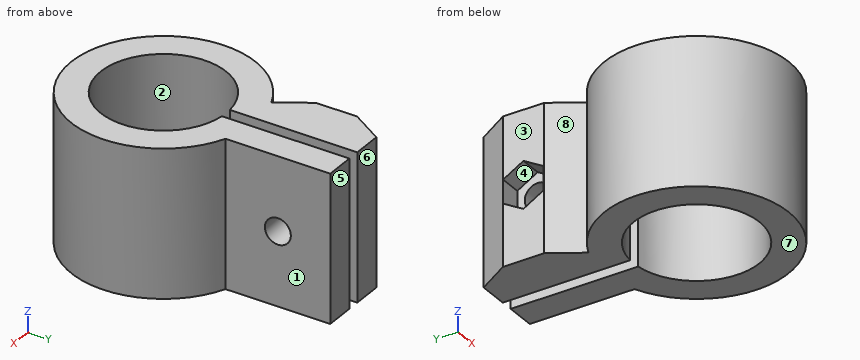
```python
from build123d import *

# Parameters (mm, degrees)
F1_DEPTH = 30
F3_DEPTH = 4.5
F4_R     = 2.646799
F5_DEPTH = 25.551


with BuildPart() as f1:
    # F0 (on Top) → F1 (new body)
    with BuildSketch(Plane.XY):
        with BuildLine():
            ThreePointArc((1.25, 12.738819), (0, -12.8), (-1.25, 12.738819))
            Line((-1.25, 12.738819), (-1.25, 38.745821))
            Line((-1.25, 38.745821), (-7.25, 38.745821))
            Line((-7.25, 38.745821), (-7.25, 17.345821))
            ThreePointArc((-7.25, 17.345821), (0, -18.8), (7.25, 17.345821))
            Line((7.25, 17.345821), (7.25, 38.738819))
            Line((7.25, 38.738819), (1.25, 38.738819))
            Line((1.25, 38.738819), (1.25, 12.738819))
        make_face()
        Polygon((-7.25, 17.345821), (-7.25, 38.745821), (-11.25, 32.245821), (-11.25, 23.845821), align=None)
    extrude(amount=F1_DEPTH)

    # F2 (on face) → F3 (cut)
    with BuildSketch(Plane(origin=(-11.25, 0, 0), x_dir=(0, -1, 0), z_dir=(-1, 0, 0))):
        Polygon((-32.195821, 17.396004), (-32.195821, 12.603996), (-28.045821, 10.207993), (-23.895821, 12.603996), (-23.895821, 17.396004), (-28.045821, 19.792007), align=None)
    extrude(amount=-F3_DEPTH, mode=Mode.SUBTRACT)

    # F4 (on face) → F5 (cut, through all)
    with BuildSketch(Plane(origin=(-6.75, 0, 0), x_dir=(0, -1, 0), z_dir=(-1, 0, 0))):
        with Locations((-28.045821, 15)):
            Circle(F4_R)
    extrude(amount=-F5_DEPTH, mode=Mode.SUBTRACT)


solid = f1.part
```
Geometry: final body of the model. Coordinates: model frame, mm. Face numbers are marked on the shaded views. A direction names the side the tool comes from. Round coordinates to 2 decimals unless told otherwise and drop trailing zeros. Loops run counter-clockwise (first coordinate to the right, second up) from the corner with the lowest first, then second, coordinate; pieces in that order, holes last. Notation, with made-up numbers: (-18.5, -22.5) -> (28.5, -22.5) arc R20 ccw to (28.5, -10.5) -> close; hole circle Ø7 at (-31, 67). An arc over 180 degrees is marked (long way). Use one line per item in the form item = value. Start each with the question number.
1) First-contact query: P1, Ø12, axis at x = 5.5, y = 24, coming from the -Z side; P2, Ø3, axis at x = -15, z = 19.5, coming from the -Y side; P3, Ø6.5, axis at y = 23.5, z = 13, coming from the +X side; P4, Ø1.5, axis at y = -7, z = 25.5, coming from the -X side. Flat tips, straight axial feed; report the tip coordinate or a pass-through.
2) Draft query along Y for the marked faces 6, 7 and 8. Return one class per face: released by +Y, released by -Y, zero draft, split by the parting line, or undercut.
3) Access query for the marked faces 1, 2, 3, 4 and 5. Directions: +Z, -Z, +X, -X, +Y, -Y. A direction counts if a zero-diameter tool reaches every point of the face in a straight line with its end or side. Return the directions, or none.
4) Section A-A on y = 0. Output: boundary loops of the cut face in (x, z).
5) Line query: L1, parallel to X at y = 27, z = 10; L2, parallel to X at y = 0, z = 13; L3, parallel to Y at x = -9, z = 25.25. Output: solid intervals per line, ascending.
6) Section D-D on x = 11.5. Output: boundary loops of the cut face in (y, z), then the cut area to 3 significant figures.
7) Section C-C on z = 15. Output: boundary loops of the cut face in (x, y), then the cut area to 3 significant figures.
8) Section B-B on x = -6. Output: boundary loops of the cut face in (y, z), then the cut area to 3 significant figures.
Response:
q1.P1 = 0
q1.P2 = -13.08
q1.P3 = 7.25
q1.P4 = -17.73
q2.face_6 = released by +Y
q2.face_7 = zero draft
q2.face_8 = undercut
q3.face_1 = +Z, -Z, +X, +Y
q3.face_2 = +Z, -Z
q3.face_3 = +Z, -Z, -X, +Y
q3.face_4 = -X
q3.face_5 = +Z, -Z, +X, -X, +Y
q4.outline = (-18.8, 0) -> (-12.8, 0) -> (-12.8, 30) -> (-18.8, 30) -> close; (12.8, 0) -> (18.8, 0) -> (18.8, 30) -> (12.8, 30) -> close
q5.L1 = -11.25 to -1.25, 1.25 to 7.25
q5.L2 = -18.8 to -12.8, 12.8 to 18.8
q5.L3 = -16.51 to -9.1, 9.1 to 16.51, 20.19 to 35.9
q6.outline = (-14.87, 0) -> (-5.62, 0) -> (-5.62, 30) -> (-14.87, 30) -> close; (5.62, 0) -> (14.87, 0) -> (14.87, 30) -> (5.62, 30) -> close
q6.area = 555 mm^2
q7.outline = (-11.25, 23.85) -> (-7.25, 17.35) arc R18.8 ccw (long way) to (7.25, 17.35) -> (7.25, 25.4) -> (1.25, 25.4) -> (1.25, 12.74) arc R12.8 cw (long way) to (-1.25, 12.74) -> (-1.25, 25.4) -> (-6.75, 25.4) -> (-6.75, 23.9) -> (-11.25, 23.9) -> close; (-11.25, 32.2) -> (-6.75, 32.2) -> (-6.75, 30.69) -> (-1.25, 30.69) -> (-1.25, 38.75) -> (-7.25, 38.75) -> (-11.25, 32.25) -> close; (1.25, 30.69) -> (7.25, 30.69) -> (7.25, 38.74) -> (1.25, 38.74) -> close
q7.area = 788 mm^2
q8.outline = (-17.82, 0) -> (-11.31, 0) -> (-11.31, 30) -> (-17.82, 30) -> close; (11.31, 0) -> (38.75, 0) -> (38.75, 30) -> (11.31, 30) -> close; hole circle Ø5.29 at (28.05, 15)
q8.area = 996 mm^2
